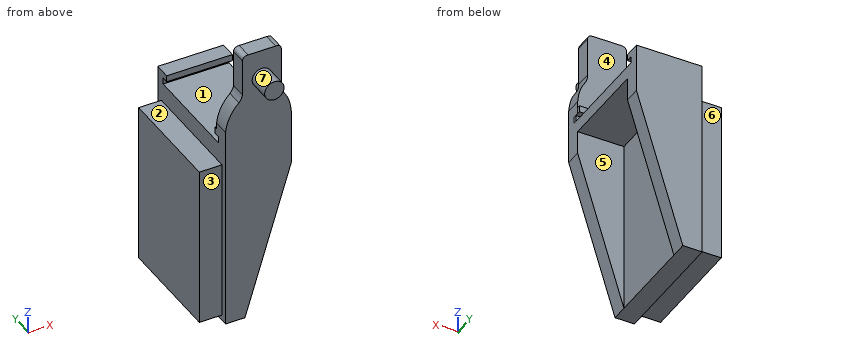
```python
from build123d import *

# Parameters (mm, degrees)
SALIENTE_EXTRUIR1_DEPTH = 19
CROQUIS2_W              = 9.87256946
CROQUIS2_H              = 14
CORTAR_EXTRUIR1_DEPTH   = 27
CROQUIS13_W             = 25.1
CROQUIS13_H             = 17
SALIENTE_EXTRUIR5_DEPTH = 3.5
CORTAR_EXTRUIR3_DEPTH   = 23
CROQUIS14_W             = 1
CROQUIS14_H             = 1
CORTAR_EXTRUIR4_DEPTH   = 23
CROQUIS15_R             = 1.5
SALIENTE_EXTRUIR6_DEPTH = 3.5
CROQUIS16_W             = 1
CROQUIS16_H             = 0.5
SALIENTE_EXTRUIR7_DEPTH = 10.165


with BuildPart() as part:
    # Croquis1 → Saliente-Extruir1 (new body)
    with BuildSketch(Plane(origin=(0, 0, 0), x_dir=(1, 0, 0), z_dir=(0, 1, 0))):
        with BuildLine():
            Line((0, 30), (0, 0))
            Line((0, 0), (0, -2))
            add(Edge.make_bspline(
                [(0, -2), (0.244064913, -4.453043064), (2.060905279, -6.231862145)],
                knots=[0, 0, 0, 1, 1, 1], degree=2))
            add(Edge.make_bspline(
                [(2.060905279, -6.231862145), (2.507004014, -6.712573557), (2.617207224, -7.344647716)],
                knots=[0, 0, 0, 1, 1, 1], degree=2))
            Line((2.617207224, -7.344647716), (2.617207224, -13.018311654))
            add(Edge.make_bspline(
                [(2.617207224, -13.018311654), (2.630895377, -13.73499915), (3.489917654, -13.737380921)],
                knots=[0, 0, 0, 1, 1, 1], degree=2))
            Line((3.489917654, -13.737380921), (7.744496795, -13.737380921))
            add(Edge.make_bspline(
                [(8.617207224, -13.018311654), (8.603519071, -13.73499915), (7.744496795, -13.737380921)],
                knots=[0, 0, 0, 1, 1, 1], degree=2))
            Line((8.617207224, -13.018311654), (8.617207224, -7.018311654))
            add(Edge.make_bspline(
                [(8.617207224, -7.018311654), (8.52941254, -6.066211773), (9.815332332, -4.707225326), (10.076873528, -2.886889338), (10.163106766, -2)],
                knots=[0, 0, 0, 0, 0.490316762, 1, 1, 1, 1], degree=3))
            Line((10.163106766, -2), (10.163106766, 0))
            Line((10.163106766, 0), (10.163106766, 6.570533479))
            Line((10.163106766, 6.570533479), (3, 30))
            Line((3, 30), (0, 30))
        make_face()
    extrude(amount=SALIENTE_EXTRUIR1_DEPTH)

    # Croquis2 → Cortar-Extruir1 (cut)
    with BuildSketch(Plane(origin=(0, 0, -30), x_dir=(-1, 0, 0), z_dir=(0, 0, -1))):
        with Locations((-7.93628473, 9.5)):
            Rectangle(CROQUIS2_W, CROQUIS2_H)
    extrude(amount=-CORTAR_EXTRUIR1_DEPTH, mode=Mode.SUBTRACT)

    # Croquis13 → Saliente-Extruir5 (add)
    with BuildSketch(Plane.ZY):
        with Locations((-16.592912937, 9.5)):
            Rectangle(CROQUIS13_W, CROQUIS13_H)
    extrude(amount=SALIENTE_EXTRUIR5_DEPTH)

    # Croquis10 → Cortar-Extruir3 (cut)
    with BuildSketch(Plane(origin=(0, 0, 0), x_dir=(0, 0, -1), z_dir=(1, 0, 0))):
        Polygon((1, 16.5), (-1, 16.5), (-1, 19), (-13.737380921, 19), (-13.737380921, 2.5), (-1, 2.5), (1, 2.5), align=None)
    extrude(amount=CORTAR_EXTRUIR3_DEPTH, mode=Mode.SUBTRACT)

    # Croquis14 → Cortar-Extruir4 (cut)
    with BuildSketch(Plane.ZY):
        with Locations((-0.5, 17)):
            Rectangle(CROQUIS14_W, CROQUIS14_H)
        with Locations((-0.5, 2)):
            Rectangle(CROQUIS14_W, CROQUIS14_H)
    extrude(amount=-CORTAR_EXTRUIR4_DEPTH, mode=Mode.SUBTRACT)

    # Croquis15 → Saliente-Extruir6 (add)
    with BuildSketch(Plane.XZ):
        with Locations((5.617207224, 9.237380921)):
            Circle(CROQUIS15_R)
    extrude(amount=SALIENTE_EXTRUIR6_DEPTH)

    # Croquis16 → Saliente-Extruir7 (add)
    with BuildSketch(Plane.ZY):
        with Locations((-0.5, 1.75)):
            Rectangle(CROQUIS16_W, CROQUIS16_H)
        with Locations((0.5, 2.75)):
            Rectangle(CROQUIS16_W, CROQUIS16_H)
    extrude(amount=-SALIENTE_EXTRUIR7_DEPTH)


solid = part.part
```
Design review of the part built by this model. Coordinates are the model's own, in mm. Face numbers are marked on the shaded views. A direction names the side the tool comes from. Give positions to 0.01 mm unless a question says otherwise; leave off trailing zeros. Order: outer loops, then holes, each group sorted by start corner. A loop starts at its lowest first (then second) coordinate and runs counter-clockwise, first axis right, second up. Notation, with made-up numbers: (34.25, 34) -> (56.25, 34) arc R28 cw to (56.25, 57) -> close; hole circle Ø4 at (-39, -33.75). An arc over 180 degrees is marked (long way). Write each question's results on one line, items separated by ' | '. Start each with the question number.
Q1. Add section A-A on y = 6. Give the boundary of the cut face in (x, z).
Q2. Add section D-D on x = -2.5. Give the boundary of the cut face in (y, z).
Q3. Mouldability with a two-part tool opening along Y and no side actions: class the marked faces 1, 2, 3 and 4 as +Y half, -Y half, draft (parallel to the pull), parting line (faces both ways), or undercut.
Q4. Add section C-C on z = -6. Give the boundary of the cut face in (x, y), and give its area (3 significant figures).
Q5. For pin 1 (8 mm diameter, centred on x = 6.5, z = 5.5, fed in from +Y); pin 2 (6 mm diameter, centred on x = 2, y = 2.5, fed in from +Z); pin 3 (8 mm diameter, centred on y = 13.5, z = -19.5, fed in from +X); pin 4 (1 mm diameter, centred on x = -2, y = 6, fed in from +Z), all flat-tipped, find the tip position at first contact; note any pin that passes through.
Q6. Machinability: for the marked faces 5, 6 and 7, which of the approach directions +Z, -Z, +X, -X, +Y, -Y give a long, thin tool a straight path to every point of the face, cutting with its end or side? Answer none if there is none.
Q7. Add section B-B on x = 6.25. Give the boundary of the cut face in (y, z), and give its area (3 significant figures).
Q8. Wall thickness on L1, parallel to Y at x = 6, z = -5; L2, parallel to Y at x = 3.25, z = 0.5; L3, parallel to Y at x = -2.75, z = -8.5: over which ranges is each line inside the solid? List them lowest first. Write a range as from..to.
Found:
1) outline: (-3.5, -29.14) -> (0, -29.14) -> (0, -30) -> (3, -30) -> (3, -3) -> (10.16, -3) -> (10.16, -1) -> (0, -1) -> (0, -4.04) -> (-3.5, -4.04) -> close
2) outline: (1, -29.14) -> (18, -29.14) -> (18, -4.04) -> (1, -4.04) -> close
3) face 1: undercut | face 2: draft | face 3: -Y half | face 4: +Y half
4) outline: (-3.5, 1) -> (0, 1) -> (0, 0) -> (10.16, 0) -> (10.16, 2.5) -> (3, 2.5) -> (3, 16.5) -> (10.16, 16.5) -> (10.16, 19) -> (0, 19) -> (0, 18) -> (-3.5, 18) -> close | area: 152 mm2
5) pin 1: stops at y = 2.5 | pin 2: stops at z = 13.74 | pin 3: stops at x = 7.02 | pin 4: stops at z = -4.04
6) face 5: -Z, +X | face 6: +Z, -Z, -X, +Y | face 7: -Y
7) outline: (-3.5, 7.88) -> (0, 7.88) -> (0, -19.37) -> (2.5, -19.37) -> (2.5, -3) -> (16.5, -3) -> (16.5, -19.37) -> (19, -19.37) -> (19, 1) -> (16.5, 1) -> (16.5, 0) -> (17.5, 0) -> (17.5, -1) -> (2, -1) -> (2, 0) -> (3, 0) -> (3, 1) -> (2.5, 1) -> (2.5, 13.74) -> (0, 13.74) -> (0, 10.6) -> (-3.5, 10.6) -> close | area: 170 mm2
8) L1: y = 0..2.5, 16.5..19 | L2: y = 0..3, 16.5..19 | L3: y = 1..18
